```python
from build123d import *

# Parameters (mm, degrees)
F1_DEPTH = 203.2


with BuildPart() as f1:
    # F0 (on Front) → F1 (new body)
    with BuildSketch(Plane.XZ):
        with BuildLine():
            Line((-42.7784153649, 23.4848271869), (-62.2295438798, 23.4436506788))
            ThreePointArc((-62.2295438798, 23.4436506788), (-77.3604186448, -4.984539736), (-52.4543076754, -25.4))
            ThreePointArc((-52.4543076754, -25.4), (-34.4937954332, -17.9605122421), (-27.0543076754, 0))
            ThreePointArc((-27.0543076754, 0), (-31.348293548, 14.1313894454), (-42.7784153649, 23.4848271869))
        make_face()
        with BuildLine():
            Line((861.8919226443, 25.399943087), (-42.7784153649, 23.4848271869))
            ThreePointArc((-42.7784153649, 23.4848271869), (-31.348293548, 14.1313894454), (-27.0543076754, 0))
            Line((-27.0543076754, 0), (836.5456923246, 0))
            ThreePointArc((836.5456923246, 0), (843.96617968, 17.9414917178), (861.8919226443, 25.399943087))
        make_face()
        with BuildLine():
            ThreePointArc((-27.0543076754, 0), (-34.4937954332, -17.9605122421), (-52.4543076754, -25.4))
            Line((-52.4543076754, -25.4), (861.9456923246, -25.4))
            ThreePointArc((861.9456923246, -25.4), (843.9851800825, -17.9605122421), (836.5456923246, 0))
            Line((836.5456923246, 0), (-27.0543076754, 0))
        make_face()
        with BuildLine():
            ThreePointArc((887.3456923246, 0), (879.8871840424, 17.9795126447), (861.8919226443, 25.399943087))
            Line((861.8919226443, 25.399943087), (862.7891166971, -25.3859928962))
            ThreePointArc((862.7891166971, -25.3859928962), (880.2019649324, -17.659799276), (887.3456923246, 0))
        make_face()
        with BuildLine():
            ThreePointArc((836.5456923246, 0), (843.9851800825, -17.9605122421), (861.9456923246, -25.4))
            ThreePointArc((861.9456923246, -25.4), (862.3674626623, -25.3964979826), (862.7891166971, -25.3859928962))
            Line((862.7891166971, -25.3859928962), (861.8919226443, 25.399943087))
            ThreePointArc((861.8919226443, 25.399943087), (843.96617968, 17.9414917178), (836.5456923246, 0))
        make_face()
    extrude(amount=F1_DEPTH)


solid = f1.part
```
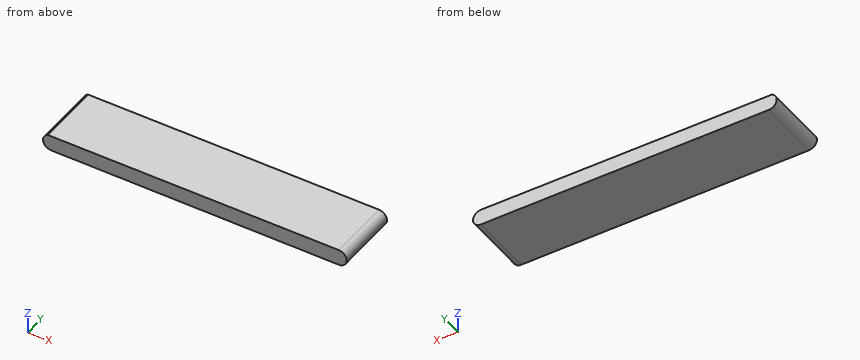
Here's how the part is built. I have some questions about the finished solid (model axes, mm). Coordinates: 2 decimals unless noted, no trailing zeros. Loops run counter-clockwise (first coordinate to the right, second up) from the corner with the lowest first, then second, coordinate; pieces in that order, holes last. Notation, with made-up numbers: (27.5, 13) -> (77.5, 13) arc R24 cw to (77.5, 41) -> close; hole circle Ø9 at (-3.75, -25). An arc over 180 degrees is marked (long way). Return JSON: item names as keys, results as strings.
1) If we section it at B-B, the plane x = 211: Write out the boundary of the cut face in (y, z), then the cut area to 3 significant figures.
Results below:
{"outline": "(-203.2, -25.4) -> (0, -25.4) -> (0, 24.02) -> (-203.2, 24.02) -> close", "area": "10,000 mm²"}
2) I need wall thicknesses on line 1 (X direction, y = -67.5, z = 1); line 2 (X direction, y = -103, z = 3); line 3 (Z direction, x = 338, y = -116.5). Which ranges of each line are inside material? Lowest first, please. Write a range as from..to.
Results below:
{"line 1": "-77.83..887.33", "line 2": "-77.68..887.17", "line 3": "-25.4..24.29"}
3) If we section it at A-A, the plane y = -105: Write out the boundary of the cut face in (x, z).
Results below:
{"outline": "(-62.23, 23.44) arc R25.4 ccw to (-52.45, -25.4) -> (861.95, -25.4) arc R25.4 ccw to (861.89, 25.4) -> close"}
4) Will these pins go through, and if not, where does the flat tip stop? pin 1 (6 mm diameter, centred on x = 395, y = -93, fed in from +Z); pin 2 (2 mm diameter, centred on y = -40.5, z = 11, fed in from +X); pin 3 (5 mm diameter, centred on y = -77.5, z = -8.5, fed in from +X); pin 4 (1 mm diameter, centred on x = 758, z = 2, fed in from +Y).
Results below:
{"pin 1": "z = 24.42", "pin 2": "x = 885.29", "pin 3": "x = 886.63", "pin 4": "y = 0"}
